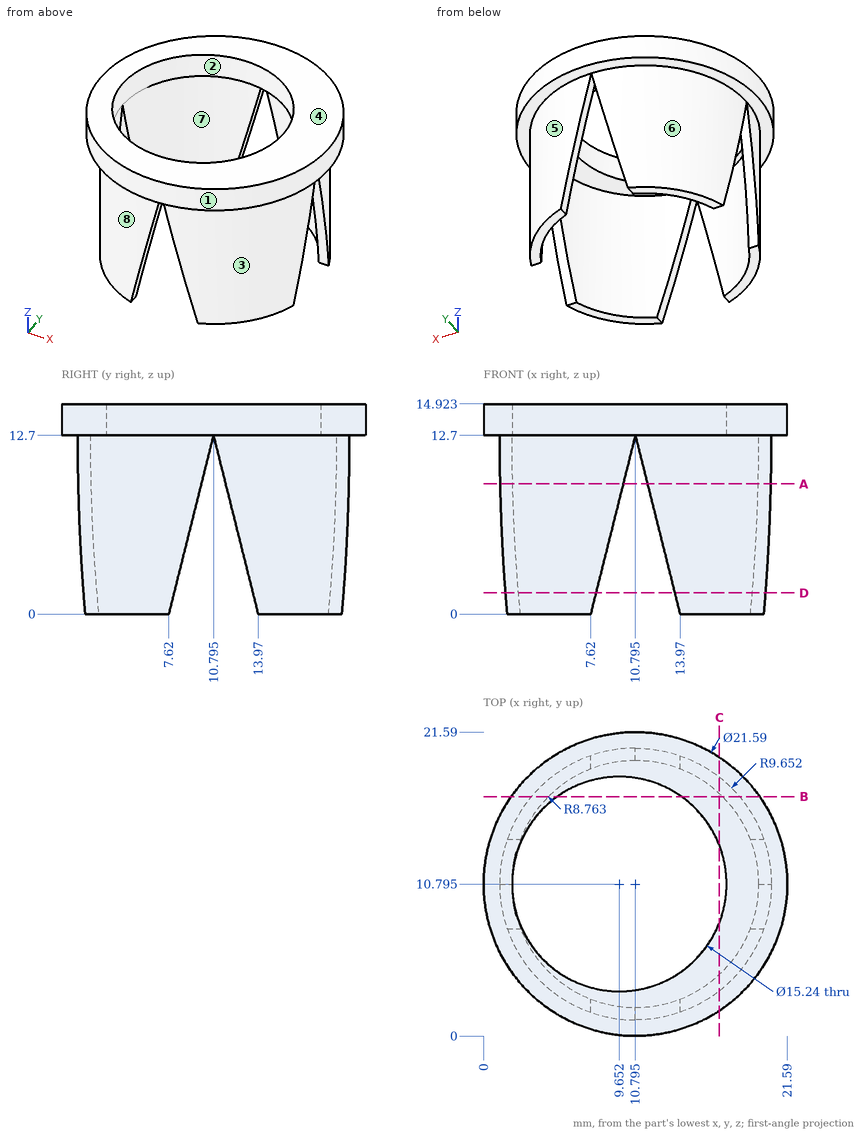
Answer from the drawing. Dimensions are ordinates in mm from the lowest x, y and z of the part. A direction names the side the tool comes from. Round coordinates to 2 decimals unless told otherwise and drop trailing zeros. Order: outer loops, then holes, each group sorted by start corner. A loop starts at its lowest first (then second) coordinate and runs counter-clockwise, first axis right, second up.
1) Straight lines are drawn through the part: L1, parallel to Z at x = 1.5, y = 6.25; L2, parallel to X at y = 11.5, z = 11.5; L3, parallel to X at y = 5.25, z = 13.5 (1 decimal). For each, find the intervals that lie inside material, in ascending order.
2) The part is cut by section D-D on z = 1.5. Write down the section's boundary in (x, y) (1 decimal).
3) The part is cut by section A-A on z = 9.25. Write down the section's boundary in (x, y) (1 decimal).
4) The mould has two halves that part along Y. Classify the marked faces 1, 2 and 3: released by +Y, released by -Y, zero draft, split by the parting line, or undercut.
5) For the marked faces 4, 5, 6, 7 and 8, determine the directions among +Z, -Z, +X, -X, +Y, -Y from which every point of the face is accessible in a straight line to the end or side of a thin tool.
6) The part is cut by section B-B on y = 17. Write down the section's boundary in (x, z) (1 decimal).
7) The part is cut by section C-C on x = 16.75. Write down the section's boundary in (y, z).
8) A flat-ended cylindrical pin translates along its axis: pin 1 (1.5 mm diameter, centred on x = 14.5, z = 8.5, fed in from -Y). Find the tip coordinate at first contact, or state that the pin passes through.
Resolved:
1. L1: z = 12.7 to 14.92
1. L2: x = 1.17 to 2.06, 19.53 to 20.42
1. L3: x = 1.5 to 4.4, 14.9 to 20.1
2. outline: (1.6, 8) arc R9.7 ccw to (8, 1.6) - (8, 2.5) arc R8.8 cw to (2.5, 8) - close; (1.6, 13.6) - (2.5, 13.6) arc R8.8 cw to (8, 19.1) - (8, 20) arc R9.7 ccw to start; (13.6, 1.6) arc R9.7 ccw to (20, 8) - (19.1, 8) arc R8.8 cw to (13.6, 2.5) - close; (13.6, 19.1) arc R8.8 cw to (19.1, 13.6) - (20, 13.6) arc R9.7 ccw to (13.6, 20) - close
3. outline: (1.2, 9.9) arc R9.7 ccw to (9.9, 1.2) - (9.9, 2.1) arc R8.8 cw to (2.1, 9.9) - close; (1.2, 11.7) - (2.1, 11.7) arc R8.8 cw to (9.9, 19.5) - (9.9, 20.4) arc R9.7 ccw to start; (11.7, 1.2) arc R9.7 ccw to (20.4, 9.9) - (19.5, 9.9) arc R8.8 cw to (11.7, 2.1) - close; (11.7, 19.5) arc R8.8 cw to (19.5, 11.7) - (20.4, 11.7) arc R9.7 ccw to (11.7, 20.4) - close
4. face 1: split by the parting line
4. face 2: undercut
4. face 3: released by -Y
5. face 4: +Z, +X, -X, +Y, -Y
5. face 5: -Z, +X, +Y
5. face 6: -Z, -X, +Y
5. face 7: -Z
5. face 8: -Z, -X, -Y
6. outline: (2, 12.7) - (3.4, 12.7) - (3.4, 0) - (4.6, 0) - (4.6, 12.7) - (5.2, 12.7) - (5.2, 14.9) - (2, 14.9) - close; (14.1, 12.7) - (17, 12.7) - (17, 0) - (18.2, 0) - (18.2, 12.7) - (19.6, 12.7) - (19.6, 14.9) - (14.1, 14.9) - close
7. outline: (1.79, 12.7) - (3.2, 12.7) - (3.2, 0) - (4.37, 0) - (4.37, 12.7) - (8.02, 12.7) - (8.02, 14.92) - (1.79, 14.92) - close; (13.57, 12.7) - (17.22, 12.7) - (17.22, 0) - (18.39, 0) - (18.39, 12.7) - (19.8, 12.7) - (19.8, 14.92) - (13.57, 14.92) - close
8. pin 1: stops at y = 1.61
